from build123d import *

# Parameters (mm, degrees)
F1_DEPTH = 27.94
F2_R     = 11.43
F3_DEPTH = 2.0066
F4_R     = 6.35
F5_DEPTH = 25.4


with BuildPart() as f1:
    # F0 (on Right) → F1 (new body)
    with BuildSketch(Plane.YZ):
        Polygon((0, 12.7), (0, 0), (50.8, 0), (76.2, 12.7), align=None)
    extrude(amount=F1_DEPTH)

    # F2 (on face) → F3 (cut)
    with BuildSketch(Plane.XY.offset(12.7)):
        with Locations((13.97, 36.576)):
            Circle(F2_R)
    extrude(amount=-F3_DEPTH, mode=Mode.SUBTRACT)

    # F4 (on face) → F5 (cut)
    with BuildSketch(Plane.XY.offset(12.7)):
        with Locations((0, 36.380674)):
            Circle(F4_R)
    extrude(amount=-F5_DEPTH, mode=Mode.SUBTRACT)


solid = f1.part
CAD build for the part. Positions are in the model's coordinates, mm. A direction names the side the tool comes from. Round coordinates to 2 decimals unless told otherwise and drop trailing zeros. Write each loop counter-clockwise with the first axis right and the second up, starting at its lowest first coordinate (ties: lowest second). Pieces come first, ordered by that corner, then holes.
(1) Slice it at D-D, the plane x = 13.97. Write the cut outline in (y, z).
(2) 3-axis set-ups, long thin cutter, end or side, ignore diameter. For faces 4 (the face through (14, 37, 10.693)), 5 (the face through (14, 25, 0)): which of +Z, -Z, +X, -X, +Y, -Y reach the whole face in a straight line?
(3) Slice it at B-B, the plane y = 45. Write the cut outline in (x, z), and give its area (3 significant figures).
(4) Drop flat-ended pins along their axis: P1, Ø3, axis at y = 37, z = 4, coming from the -X side; P2, Ø3, axis at x = 17.5, y = 32, coming from the +Z side; P3, Ø6, axis at y = 35.5, z = 11.5, coming from the -X side. Give the stop position or say it passes through.
(5) Mould opens along Y. For faces 1 (the face through (13.77, 63.32, 6.26)), 2 (the face through (0, 56, 8)), 3 (the face through (25.397, 36.307, 11.711)) say: pulls with the +Y half, pulls with the -Y half, needs draft (parallel to the pull), parting line crosses it, or undercut.
(6) Probe line 1 along Z through (x, y) = (6, 29); line 2 along Y through (x, z) = (5.75, 12); line 3 along Y through (x, z) = (2.5, 3.25). List the from-to ranges inside material, lowest first.
(7) Slice it at A-A, the plane x = 5. Write the cut outline in (y, z).
(8) Slice it at C-C, the plane z = 1. Write the cut outline in (x, y).
From the geometry:
1. outline: (0, 0) - (50.8, 0) - (76.2, 12.7) - (48.01, 12.7) - (48.01, 10.69) - (25.15, 10.69) - (25.15, 12.7) - (0, 12.7) - close
2. face 4: +Z
2. face 5: -Z, +X, -X, +Y, -Y
3. outline: (0, 0) - (27.94, 0) - (27.94, 12.7) - (21.7, 12.7) - (21.7, 10.69) - (6.24, 10.69) - (6.24, 12.7) - (0, 12.7) - close
3. area: 324 mm2
4. P1: stops at x = 5.99
4. P2: stops at z = 10.69
4. P3: stops at x = 5.11
5. face 1: pulls with the +Y half
5. face 2: needs draft
5. face 3: undercut
6. line 1: z = 0 to 10.69
6. line 2: y = 0 to 28.63, 44.52 to 74.8
6. line 3: y = 0 to 30.54, 42.22 to 57.3
7. outline: (0, 0) - (32.47, 0) - (32.47, 10.69) - (29.49, 10.69) - (29.49, 12.7) - (0, 12.7) - close; (40.3, 0) - (50.8, 0) - (76.2, 12.7) - (43.66, 12.7) - (43.66, 10.69) - (40.3, 10.69) - close
8. outline: (0, 0) - (27.94, 0) - (27.94, 52.8) - (0, 52.8) - (0, 42.73) arc R6.35 cw to (0, 30.03) - close
